The listing builds one solid part. Answer for the finished solid, in the listing's coordinates (mm). Face numbers are marked on the shaded views. A direction names the side the tool comes from. Round coordinates to 2 decimals unless told otherwise and drop trailing zeros. Order: outer loops, then holes, each group sorted by start corner. A loop starts at its lowest first (then second) coordinate and runs counter-clockwise, first axis right, second up. Notation, with made-up numbers: (73, 24) - (102, 24) arc R18 cw to (102, 40) - close; hole circle Ø2 at (2, 9.25). An arc over 180 degrees is marked (long way). Write item = value, one per line.
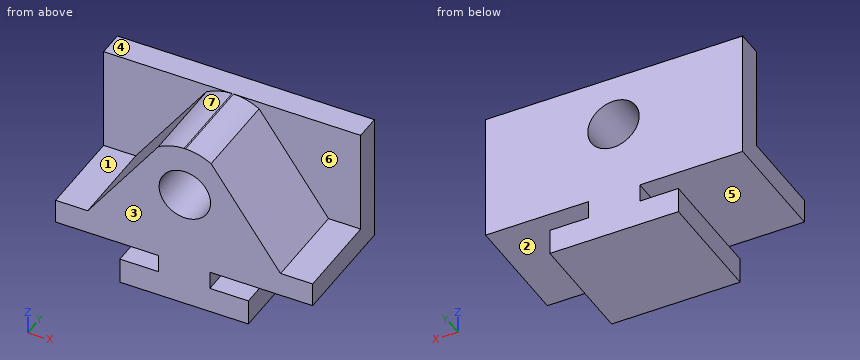
from build123d import *

# Parameters (mm, degrees)
F0_W     = 15.875
F0_H     = 44.45
F0_W_2   = 95.25
F1_DEPTH = 85.09
F3_DEPTH = 44.45
F2_R     = 12.7
F4_DEPTH = 57.151


with BuildPart() as f1:
    # F0 (on Top) → F1 (new body)
    with BuildSketch(Plane.XY):
        with Locations((7.9375, 22.225)):
            Rectangle(F0_W, F0_H)
        with Locations((63.5, 22.225)):
            Rectangle(F0_W_2, F0_H)
        Polygon((0, 57.15), (0, 44.45), (15.875, 44.45), (111.125, 44.45), (127, 44.45), (127, 57.15), align=None)
        with Locations((119.0625, 22.225)):
            Rectangle(F0_W, F0_H)
    extrude(amount=F1_DEPTH)

    # F2 (on face) → F3 (cut)
    with BuildSketch(Plane.XZ):
        with BuildLine():
            Line((63.5, 85.09), (0, 85.09))
            Line((0, 85.09), (0, 33.536568))
            Line((0, 33.536568), (15.875, 33.536568))
            Line((15.875, 33.536568), (50.849151, 81.520875))
            ThreePointArc((50.849151, 81.520875), (56.939695, 84.137978), (63.5, 85.09))
        make_face()
        with BuildLine():
            Line((127, 85.09), (64.172919, 85.09))
            ThreePointArc((64.172919, 85.09), (70.733224, 84.137978), (76.823767, 81.520875))
            Line((76.823767, 81.520875), (111.125, 33.536568))
            Line((111.125, 33.536568), (127, 33.536568))
            Line((127, 33.536568), (127, 85.09))
        make_face()
    extrude(amount=-F3_DEPTH, mode=Mode.SUBTRACT)

    # F2 (on face) → F4 (cut, through all)
    with BuildSketch(Plane.XZ):
        Polygon((127, 0), (127, 21.59), (76.2, 21.59), (76.2, 12.7), (95.25, 12.7), (95.25, 0), align=None)
        Polygon((50.8, 21.59), (0, 21.59), (0, 0), (31.75, 0), (31.75, 12.7), (50.8, 12.7), align=None)
        with Locations((63.836459, 59.692229)):
            Circle(F2_R)
    extrude(amount=-F4_DEPTH, mode=Mode.SUBTRACT)


solid = f1.part
Q1. Find the intervals of material crossed by line 1 (X direction, y = 41.5, z = 6.5); line 2 (Z direction, x = 45, y = 20); line 3 (Z direction, x = 18, y = 49), in increasing order. Write a range as from..to.
Model answer:
line_1 = 31.75..95.25
line_2 = 0..12.7, 21.59..73.5
line_3 = 21.59..85.09
Q2. Section A-A on z = 65 is taken. Determine the outline of the cut face in (x, y).
Model answer:
outline = (0, 44.45) - (38.81, 44.45) - (38.81, 0) - (52.3, 0) - (52.3, 57.15) - (0, 57.15) - close; (75.37, 0) - (88.63, 0) - (88.63, 44.45) - (127, 44.45) - (127, 57.15) - (75.37, 57.15) - close
Q3. Flat-ended cylindrical pins translate along their axes: P1, Ø4, axis at y = 33, z = 8.5, coming from the -X side; P2, Ø5, axis at x = 121.5, y = 14.5, coming from the +Z side; P3, Ø3, axis at x = 76.5, y = 25, coming from the +Z side. Find the tip coordinate at first contact, or state that the pin passes through.
Model answer:
P1 = 31.75
P2 = 33.54
P3 = 82.51
Q4. For the marked faces 4, 5, 6 and 7, determine the directions among +Z, -Z, +X, -X, +Y, -Y from which every point of the face is accessible in a straight line to the end or side of a thin tool.
Model answer:
face_4 = +Z, +X, -X, +Y, -Y
face_5 = -X, +Y, -Y
face_6 = +Z, +X, -Y
face_7 = +Z, -X, -Y
Q5. Determine the mould class of the marked faces 1, 2 and 3 for opening direction Z: released by +Z, released by -Z, zero draft, split by the parting line, or undercut.
Model answer:
face_1 = released by +Z
face_2 = undercut
face_3 = zero draft
Q6. Section D-D on z = 45 is taken. Determine the outline of the cut face in (x, y).
Model answer:
outline = (0, 44.45) - (24.23, 44.45) - (24.23, 0) - (102.93, 0) - (102.93, 44.45) - (127, 44.45) - (127, 57.15) - (0, 57.15) - close
Q7. Section C-C on y = 20 is taken. Determine the outline of the cut face in (x, z) (3 decimals).
Model answer:
outline = (0, 21.59) - (50.8, 21.59) - (50.8, 12.7) - (31.75, 12.7) - (31.75, 0) - (95.25, 0) - (95.25, 12.7) - (76.2, 12.7) - (76.2, 21.59) - (127, 21.59) - (127, 33.537) - (111.125, 33.537) - (76.824, 81.521) arc R25.4 ccw to (64.173, 85.09) - (63.5, 85.09) arc R25.4 ccw to (50.849, 81.521) - (15.875, 33.537) - (0, 33.537) - close; hole circle Ø25.4 at (63.836, 59.692)
Q8. Section B-B on x = 79 is taken. Determine the outline of the cut face in (y, z).
Model answer:
outline = (0, 0) - (57.15, 0) - (57.15, 12.7) - (0, 12.7) - close; (0, 21.59) - (57.15, 21.59) - (57.15, 85.09) - (44.45, 85.09) - (44.45, 78.48) - (0, 78.48) - close
